Input: part model. Units: mm. Frame: model coordinates. Face numbers are marked on the shaded views. A direction names the side the tool comes from. Coordinates: 2 decimals unless noted, no trailing zeros. Loops run counter-clockwise (first coordinate to the right, second up) from the corner with the lowest first, then second, coordinate; pieces in that order, holes last.
Autodesk Inventor part; units mm, degrees
ref_plane "YZ Plane" through (0, 0, 0) normal (1, 0, 0) x (0, 1, 0)
ref_plane "XZ Plane" through (0, 0, 0) normal (0, 1, 0) x (-1, 0, 0)
ref_plane "XY Plane" through (0, 0, 0) normal (0, 0, 1) x (1, 0, 0)
sketch "Sketch1" plane through (0, 0, 0) normal (0, 1, 0) x (-1, 0, 0)
  line L0 (0, 0) -> (40, 0)
  line L1 (40, 0) -> (40, -49)
  line L2 (40, -49) -> (0, -49)
  line L3 (0, -49) -> (0, 0)
  dimension "d0" = 40
  dimension "d1" = 49
extrude "Extrusion1" add sketch "Sketch1" along normal blind 24
sketch "Sketch2" plane through (0, 24, 0) normal (0, 1, 0) x (1, 0, 0)
  line L0 (0, 0) -> (0, 49)
  line L1 (0, 49) -> (-40, 49)
  line L2 (0, 0) -> (-2, 0)
  line L3 (-2, 0) -> (-2, 49)
  line L4 (-2, 49) -> (0, 49)
  line L5 (0, 49) -> (0, 0)
  line L6 (-40, 49) -> (-40, 0)
  line L7 (-40, 0) -> (-38, 0)
  line L8 (-38, 0) -> (-38, 49)
  line L9 (-38, 49) -> (-40, 49)
  line L10 (-40, 49) -> (-40, 0)
  line L11 (0, 0) -> (-40, 0)
  line L12 (-40, 0) -> (-40, 2)
  line L13 (-40, 2) -> (0, 2)
  line L14 (0, 2) -> (0, 0)
  line L15 (0, 49) -> (-40, 49)
  line L16 (-40, 49) -> (-40, 47)
  line L17 (-40, 47) -> (0, 47)
  line L18 (0, 47) -> (0, 49)
  line L19 (-2, 47) -> (-38, 47)
  line L20 (-38, 47) -> (-38, 2)
  line L21 (-38, 2) -> (-2, 2)
  line L22 (-2, 2) -> (-2, 47)
  point P0 (-38, 47)
  dimension "d4" = 2
  dimension "d5" = 2
  dimension "d6" = 2
  dimension "d7" = 2
extrude "Extrusion2" cut sketch "Sketch2" against normal blind 21.75 contours L13 L8 L17 L3
sketch "Sketch3" plane through (-40, 0, 0) normal (0, 0, 1) x (1, 0, 0)
  line L0 (0, 24) -> (40, 24)
  line L1 (0, 0) -> (40, 0)
  line L2 (0, 24) -> (8, 24)
  line L3 (8, 24) -> (8, 0)
  line L4 (8, 0) -> (0, 0)
  line L5 (0, 0) -> (0, 24)
  line L6 (0, 0) -> (0, 24)
  line L7 (40, 0) -> (40, 24)
  line L8 (0, 0) -> (40, 0)
  line L9 (40, 0) -> (40, 8)
  line L10 (40, 8) -> (0, 8)
  line L11 (0, 8) -> (0, 0)
  line L12 (38, 24) -> (2, 24)
  line L13 (40, 0) -> (32, 0)
  line L14 (32, 0) -> (32, 24)
  line L15 (32, 24) -> (40, 24)
  line L16 (40, 24) -> (40, 0)
  line L17 (8, 24) -> (32, 24)
  line L18 (32, 24) -> (32, 8)
  line L19 (32, 8) -> (8, 8)
  line L20 (8, 8) -> (8, 24)
  point P0 (8, 8)
  dimension "d10" = 8
  dimension "d11" = 8
  dimension "d12" = 8
extrude "Extrusion3" cut sketch "Sketch3" against normal blind 21 contours L0 L14 L10 L3
fillet "Fillet1" radius 5 2 edges at (-32, 8, -1) (-8, 8, -1)
sketch "Sketch4" plane through (-40, 0, 0) normal (0, 0, 1) x (1, 0, 0)
  line L0 (0, 0) -> (0, 24)
  line L1 (8, 13) -> (8, 24)
  line L2 (0, 24) -> (8, 24)
  line L3 (8, 24) -> (8, 20)
  line L4 (8, 20) -> (0, 20)
  line L5 (0, 20) -> (0, 24)
  line L6 (32, 24) -> (40, 24)
  line L7 (32, 13) -> (32, 24)
  line L8 (40, 24) -> (32, 24)
  line L9 (32, 24) -> (32, 20)
  line L10 (32, 20) -> (40, 20)
  line L11 (40, 20) -> (40, 24)
  point P0 (40, 0)
  point P1 (0, 20)
  dimension "d16" = 4
  dimension "d17" = 4
extrude "Extrusion4" add sketch "Sketch4" along normal blind 5
sketch "Sketch5" plane through (0, 0, -49) normal (0, 0, -1) x (-1, 0, 0)
  line L0 (40, 0) -> (40, 24)
  line L1 (0, 24) -> (40, 24)
  line L2 (40, 24) -> (40, 20)
  line L3 (40, 20) -> (0, 20)
  line L4 (0, 20) -> (0, 24)
  point P0 (0, 0)
  dimension "d20" = 4
extrude "Extrusion5" add sketch "Sketch5" along normal blind 5
sketch "Sketch6" plane through (-2, 24, -47) normal (-1, 0, 0) x (0, 0, 1)
  line L0 (0, 0) -> (0, -21.75)
  line L1 (0, 0) -> (45, 0)
  line L2 (0, -21.75) -> (45, -21.75)
  line L3 (45, -21.75) -> (45, 0)
  line L4 (45, 0) -> (0, 0)
  line L5 (0, 0) -> (0, -21.75)
  point P0 (47, -24)
extrude "Extrusion6" cut sketch "Sketch6" along normal blind 50
sketch "Sketch10" plane through (0, 0, 0) normal (0, -1, 0) x (1, 0, 0)
  line L0 (-8, 5) -> (0, 5)
  line L1 (0, 5) -> (-4, 5)
  line L2 (-4, 5) -> (-4, 2.5)
  line L3 (-4, 2.5) -> (0, 2.5)
  line L4 (0, 2.5) -> (0, 5)
  circle A0 centre (-4, 2.5) radius 0.5
  line L5 (-40, 0) -> (-40, 5)
  line L6 (-40, 5) -> (-36, 5)
  line L7 (-36, 5) -> (-36, 2.5)
  line L8 (-36, 2.5) -> (-40, 2.5)
  line L9 (-40, 2.5) -> (-40, 5)
  circle A1 centre (-36, 2.5) radius 0.5
  line L10 (-40, 5) -> (-40, -54)
  line L11 (-40, -54) -> (-36, -54)
  line L12 (-36, -54) -> (-36, -51.5)
  line L13 (-36, -51.5) -> (-40, -51.5)
  line L14 (-40, -51.5) -> (-40, -54)
  circle A2 centre (-36, -51.5) radius 0.5
  line L15 (0, -54) -> (0, 5)
  line L16 (0, -54) -> (-4, -54)
  line L17 (-4, -54) -> (-4, -51.5)
  line L18 (-4, -51.5) -> (0, -51.5)
  line L19 (0, -51.5) -> (0, -54)
  circle A3 centre (-4, -51.5) radius 0.5
  point P0 (0, 0)
  point P1 (0, -47)
  dimension "d41" = 4
  dimension "d42" = 2.5
  dimension "d43" = 1
  dimension "d44" = 4
  dimension "d45" = 2.5
  dimension "d46" = 1
  dimension "d49" = 4
  dimension "d50" = 2.5
  dimension "d51" = 1
  dimension "d53" = 4
  dimension "d54" = 2.5
  dimension "d55" = 1
extrude "Extrusion10" cut sketch "Sketch10" against normal blind 30 contours A0 L3 L2 | L2 L3 A0 | A3 L17 L18 | L18 L17 A3 | A1 L7 L8 | L8 L7 A1 | A2 L12 L13 | L13 L12 A2
sketch "Sketch12" plane through (-40, 0, 0) normal (0, 0, 1) x (1, 0, 0)
  line L0 (40, 20) -> (36.5, 20)
  line L1 (0, 20) -> (2, 20)
  line L2 (2, 20) -> (2, 13)
  line L3 (2, 13) -> (0, 13)
  line L4 (0, 13) -> (0, 20)
  circle A0 centre (2, 13) radius 1
  point P0 (40, 0)
  dimension "d76" = 2
  dimension "d77" = 7
  dimension "d78" = 2
extrude "Extrusion12" cut sketch "Sketch12" against normal blind 5 contours A0 L3 L2 | L2 L3 A0
sketch "Sketch14" plane through (0, 0, -49) normal (0, 0, -1) x (-1, 0, 0)
  line L0 (0, 0) -> (40, 0)
  line L1 (40, 0) -> (38, 0)
  line L2 (38, 0) -> (38, 7)
  line L3 (38, 7) -> (40, 7)
  line L4 (40, 7) -> (40, 0)
  circle A0 centre (38, 7) radius 1
  dimension "d79" = 2
  dimension "d80" = 7
  dimension "d81" = 2
extrude "Extrusion14" cut sketch "Sketch14" against normal blind 5 contours A0 L3 L2 | L2 L3 A0
sketch "Sketch15" plane through (-40, 0, -49) normal (-1, 0, 0) x (0, 0, 1)
  point P0 (49, 0)
properties part number "encaixe2 mouse"
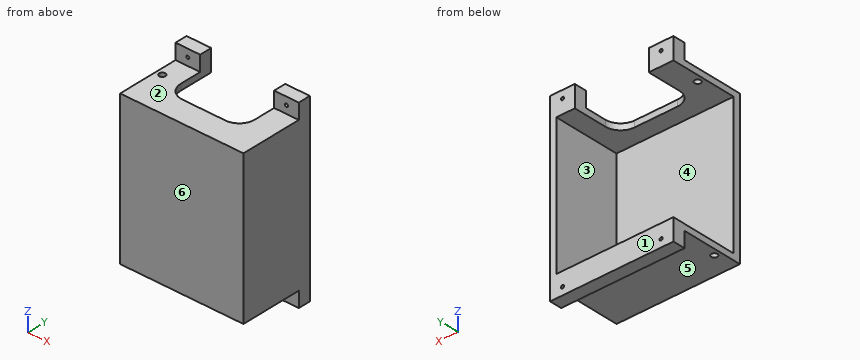
Item 1: Contact query for flat-ended pins moving along their axis: P1, Ø5, axis at x = -10, z = -15.5, coming from the +Y side; P2, Ø1.6, axis at x = -20.5, z = -1, coming from the +Y side; P3, Ø1, axis at x = -34.5, z = -36.5, coming from the -Y side; P4, Ø10, axis at x = -26, y = 9, coming from the -Z side. Output: stop coordinate, or through.
Result:
P1: stops at y = 2.25
P2: stops at y = 8
P3: stops at y = 0
P4: stops at z = -49
Item 2: Section query D-D (z = -13). Output: boundary loops of the cut face in (x, y), then the cut area to 4 significant figures.
Result:
outline: (-40, 0) - (0, 0) - (0, 24) - (-2, 24) - (-2, 2.25) - (-40, 2.25) - close
area: 133.5 mm2
Item 3: Section query A-A (x = -38). Output: boundary loops of the cut face in (y, z), then the cut area to 3 significant figures.
Result:
outline: (0, -49) - (6, -49) - (6, -47) - (2.25, -47) - (2.25, -2) - (12, -2) - (12, 0) - (0, 0) - close; (8, -49) - (20, -49) - (20, -54) - (24, -54) - (24, -47) - (8, -47) - close; (14, -2) - (24, -2) - (24, 5) - (20, 5) - (20, 0) - (14, 0) - close
area: 229 mm2
Item 4: Line query: L1, parallel to X at y = 21.9, z = -51.5; L2, parallel to Z at x = -36, y = 20.9; L3, parallel to X at y = 13, z = -1.05. Output: solid intervals per line, ascending.
Result:
L1: x = -40 to -36.5, -35.5 to -4.5, -3.5 to 0
L2: z = -54 to -52, -51 to -47, -2 to 2, 3 to 5
L3: x = -40 to -39, -37 to -32, -8 to 0
Item 5: Section query C-C (x = -22.5). Output: boundary loops of the cut face in (y, z).
Result:
outline: (0, -49) - (20, -49) - (20, -54) - (24, -54) - (24, -47) - (2.25, -47) - (2.25, -2) - (8, -2) - (8, 0) - (0, 0) - close
Item 6: Reachability of the marked faces 1, 2 and 3 from +Z, -Z, +X, -X, +Y, -Y: full face, straight path, thin tool, end or side. Return the list, or none.
Result:
face 1: +Z, -Z, +X, -X, +Y
face 2: +Z, +X, -X, -Y
face 3: -X, +Y
Item 7: Section query B-B (y = 7). Output: boundary loops of the cut face in (x, z), then the cut area to 3 significant figures.
Result:
outline: (-40, -49) - (-39, -49) - (-39, -47) - (-40, -47) - close; (-40, -2) - (-2, -2) - (-2, -47) - (-37, -47) - (-37, -49) - (0, -49) - (0, 0) - (-40, 0) - close
area: 246 mm2
Item 8: Mould query, pull axis Z, two halves, no side actions, for the marked faces 4, 5 and 6. Classes: +Z half, -Z half, draft (parallel to the pull), parting line (faces both ways), or undercut.
Result:
face 4: undercut
face 5: -Z half
face 6: draft
